```python
from build123d import *

# Parameters (mm, degrees)
F0_W     = 101.6
F0_H     = 101.6
F1_DEPTH = 25.4
F4_W     = 25.4
F4_H     = 50.8
F2_W     = 76.2
F2_H     = 76.2


with BuildPart() as f1:
    # F0 (on Top) → F1 (new body)
    with BuildSketch(Plane.XY):
        with Locations((50.8, 50.8)):
            Rectangle(F0_W, F0_H)
    extrude(amount=F1_DEPTH)

    # F4 (on offset) → F5 section 0
    with BuildSketch(Plane.XY.offset(152.4)):
        with Locations((50.8, 76.2)):
            Rectangle(F4_W, F4_H)
    # F2 (on face) → F5 section 1
    with BuildSketch(Plane.XY.offset(25.4)):
        with Locations((50.8, 63.5)):
            Rectangle(F2_W, F2_H)
    loft()


solid = f1.part
```
Could you check a few things on this model? Use its own coordinates, in mm. A direction names the side the tool comes from. Round coordinates to 2 decimals unless told otherwise and drop trailing zeros. Loops run counter-clockwise (first coordinate to the right, second up) from the corner with the lowest first, then second, coordinate; pieces in that order, holes last. Notation, with made-up numbers: (60.5, -31) -> (88.5, -31) arc R16 cw to (88.5, -7) -> close; hole circle Ø5 at (86, -2.5). An arc over 180 degrees is marked (long way). Put each result on its own line as item: value.
Q1. I want a section at A-A on y = 8. Write out the boundary of the cut face in (x, z), and give its area (3 significant figures).
Checks:
outline: (0, 0) -> (101.6, 0) -> (101.6, 25.4) -> (0, 25.4) -> close
area: 2,580 mm2
Q2. Which directions (+Z, -Z, +X, -X, +Y, -Y) give clear straight access to the entire face, cutting with the end or side of a thin tool? Please do faces 1 (the flat face through (50, 101.6, 58)), 2 (the flat face through (50, 18, 25.4)).
Checks:
face 1: +Z, -Z, +X, -X, +Y
face 2: +Z, -Y
Q3. For pin 1 Ø12 at (x, z) = (56.5, 134.5) entering from -Y; pin 2 Ø12 at (x, z) = (12.5, 82) entering from -Y; pin 3 Ø6 at (x, z) = (26.5, 65) entering from -Y; pin 4 Ø2 at (x, z) = (33, 128) entering from -Y, each with a flat end and sliding along its axis, tell me the tip position at first contact or that it passes through.
Checks:
pin 1: y = 46.02
pin 2: through
pin 3: y = 32.72
pin 4: y = 45.72
Q4. Please list where these lines run through material, in increasing order: line 1 (Z direction, x = 71.5, y = 22); line 2 (X direction, y = 95.5, z = 74.5); line 3 (X direction, y = 84, z = 70). Write a range as from..to.
Checks:
line 1: 0..25.4
line 2: 22.52..79.08
line 3: 21.62..79.98
